Here's how the part is built. I have some questions about the finished solid (model axes, mm). Face numbers are marked on the shaded views. A direction names the side the tool comes from. Give positions to 0.01 mm unless a question says otherwise; leave off trailing zeros. Loops run counter-clockwise (first coordinate to the right, second up) from the corner with the lowest first, then second, coordinate; pieces in that order, holes last. Notation, with made-up numbers: (36, 57.25) - (43, 57.25) arc R24 ccw to (43, 93.25) - close; hole circle Ø9 at (-37, 23.25). An arc over 180 degrees is marked (long way). Use one line per item in the form item = value.
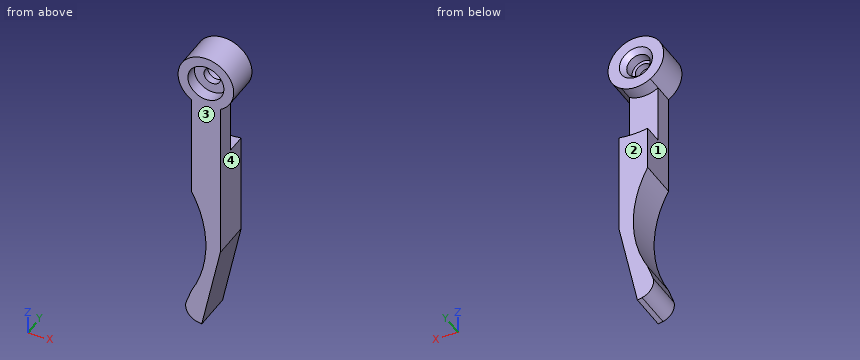
from build123d import *

# Parameters (mm, degrees)
BOSS_EXTRU_1_DEPTH      = 8
ESQUISSE2_R             = 2.45
ENL_V_MAT_EXTRU_1_DEPTH = 4
ENL_V_MAT_EXTRU_2_REACH = 59.094
ESQUISSE3_R             = 1.75
ESQUISSE4_R             = 3.75
ENL_V_MAT_EXTRU_3_DEPTH = 2.5
ENL_V_MAT_EXTRU_4_DEPTH = 4
ESQUISSE7_R             = 5.8
ENL_V_MAT_EXTRU_5_DEPTH = 1
CHANFREIN1_SIZE         = 1


with BuildPart() as part:
    # Esquisse1 → Boss.-Extru.1 (new body)
    with BuildSketch(Plane(origin=(0, 0, 0), x_dir=(1, 0, 0), z_dir=(0, 1, 0))):
        with BuildLine():
            Line((-3, 26.381049961), (-3, 4.963869458))
            ThreePointArc((-3, 4.963869458), (0, -5.8), (3, 4.963869458))
            Line((3, 4.963869458), (3, 38.463869458))
            Line((3, 38.463869458), (-0.867157449, 56.657414832))
            Line((-0.867157449, 56.657414832), (-1.84530505, 56.449503141))
            ThreePointArc((-1.84530505, 56.449503141), (-3.756758837, 55.119060789), (-4.140414176, 52.821988519))
            Line((-4.140414176, 52.821988519), (-3, 49.618950039))
            ThreePointArc((-3, 49.618950039), (0, 38), (-3, 26.381049961))
        make_face()
    extrude(amount=BOSS_EXTRU_1_DEPTH)

    # Esquisse2 → Enlèv. mat.-Extru.1 (cut)
    with BuildSketch(Plane(origin=(0, 8, 0), x_dir=(1, 0, 0), z_dir=(0, 1, 0))):
        with Locations(Location((0, 0, 0), (0, 0, 270))):
            Circle(ESQUISSE2_R)
    extrude(amount=-ENL_V_MAT_EXTRU_1_DEPTH, mode=Mode.SUBTRACT)

    # Esquisse3 → Enlèv. mat.-Extru.2 (cut, up to next)
    with BuildSketch(Plane(origin=(0, 4, 0), x_dir=(1, 0, 0), z_dir=(0, 1, 0)), mode=Mode.PRIVATE) as enl_v_mat_extru_2_sk1:
        with Locations(Location((0, 0, 0), (0, 0, 270))):
            Circle(ESQUISSE3_R)
    enl_v_mat_extru_2_tool1 = extrude(enl_v_mat_extru_2_sk1.sketch, amount=-ENL_V_MAT_EXTRU_2_REACH, mode=Mode.PRIVATE) & part.part
    add(enl_v_mat_extru_2_tool1.solids().sort_by_distance((0, 4, 0))[0], mode=Mode.SUBTRACT)

    # Esquisse4 → Enlèv. mat.-Extru.3 (cut)
    with BuildSketch(Plane.XZ):
        with Locations(Location((0, 0, 0), (0, 0, 270))):
            Circle(ESQUISSE4_R)
    extrude(amount=-ENL_V_MAT_EXTRU_3_DEPTH, mode=Mode.SUBTRACT)

    # Esquisse5 → Enlèv. mat.-Extru.4 (cut)
    with BuildSketch(Plane(origin=(0, 8, 0), x_dir=(1, 0, 0), z_dir=(0, 1, 0))):
        with BuildLine():
            Line((-3, 4.963869458), (-3, 17.24093965))
            ThreePointArc((-3, 17.24093965), (0, 17.5), (3, 17.24093965))
            Line((3, 17.24093965), (3, 4.963869458))
            ThreePointArc((3, 4.963869458), (0, 5.8), (-3, 4.963869458))
        make_face()
    extrude(amount=-ENL_V_MAT_EXTRU_4_DEPTH, mode=Mode.SUBTRACT)

    # Esquisse7 → Enlèv. mat.-Extru.5 (cut)
    with BuildSketch(Plane(origin=(0, 8, 0), x_dir=(1, 0, 0), z_dir=(0, 1, 0))):
        with Locations(Location((0, 0, 0), (0, 0, 58.852610078))):
            Circle(ESQUISSE7_R)
    extrude(amount=-ENL_V_MAT_EXTRU_5_DEPTH, mode=Mode.SUBTRACT)

    # Chanfrein1
    chanfrein1_edges = [part.edges().sort_by_distance(p)[0] for p in [
        (0, 7, -2.45),
    ]]
    chamfer(chanfrein1_edges, length=CHANFREIN1_SIZE)


solid = part.part
(1) For the marked faces 3 and 4, which set-ups out of +Z, -Z, +X, -X, +Y, -Y let a thin tool reach every point of the face, with its end or its side?
Geometry says:
face_3 = +Z, -Z, +X, -X, -Y
face_4 = -Z, +X, +Y, -Y
(2) If we section it at C-C (z = -23): List the corners of the cut face in (x, y) for me.
Geometry says:
outline = (-3, 0) - (3, 0) - (3, 8) - (-3, 8) - close
(3) Thinking about a two-plate mould opening in Z: for the marked faces 1 and 2, which applies, pulls with the +Z half, pulls with the -Z half, needs draft (parallel to the pull), parting line crosses it, or undercut?
Geometry says:
face_1 = undercut
face_2 = needs draft
(4) If we section it at B-B (z = -7): List the corners of the cut face in (x, y) for me, plus the area to 3 significant figures.
Geometry says:
outline = (-3, 0) - (3, 0) - (3, 4) - (-3, 4) - close
area = 24.0 mm²
(5) For P1, Ø1.5, axis at x = 0.5, z = -5, coming from the +Y side; P2, Ø2, axis at x = 2.5, y = 5.5, coming from the +Z side; P3, Ø4, axis at x = -1.5, z = 0, coming from the -Y side; P4, Ø2, axis at x = -4.5, z = -21, coming from the -Y side, each with a flat end and sliding along its axis, tell me the tip position at first contact or that it passes through.
Geometry says:
P1 = 7
P2 = 5.6
P3 = 2.5
P4 = through
(6) If we section it at A-A (y = 1.5): List the corners of the cut face in (x, z) for me.
Geometry says:
outline = (-4.14, -52.82) arc R3 ccw to (-1.85, -56.45) - (-0.87, -56.66) - (3, -38.46) - (3, -4.96) arc R5.8 ccw (long way) to (-3, -4.96) - (-3, -26.38) arc R24 cw to (-3, -49.62) - close; hole circle Ø7.5 at (0, 0)
(7) If I drill on probe 1 along X at (y, z) = (1.9, 0); probe 2 along X at (y, z) = (4.95, 0); probe 3 along Y at (x, z) = (1.5, -9), over which ranges is the centre line in solid material (lowest first)?
Geometry says:
probe_1 = -5.8 to -3.75, 3.75 to 5.8
probe_2 = -5.8 to -2.45, 2.45 to 5.8
probe_3 = 0 to 4
